Input: dimensioned drawing with shaded views. Units: mm. Origin: part minimum x, y, z. Give positions to 0.01 mm unless a question says otherwise; leave off trailing zeros. Order: outer loops, then holes, each group sorted by start corner. A loop starts at its lowest first (then second) coordinate and runs counter-clockwise, first axis right, second up. Notation, with made-up numbers: (70, -4.75) - (106, -4.75) arc R14 ccw to (106, 5.25) - close; hole circle Ø4 at (11.5, 39). An arc over 180 degrees is marked (long way). Use a Markdown table: item, result.
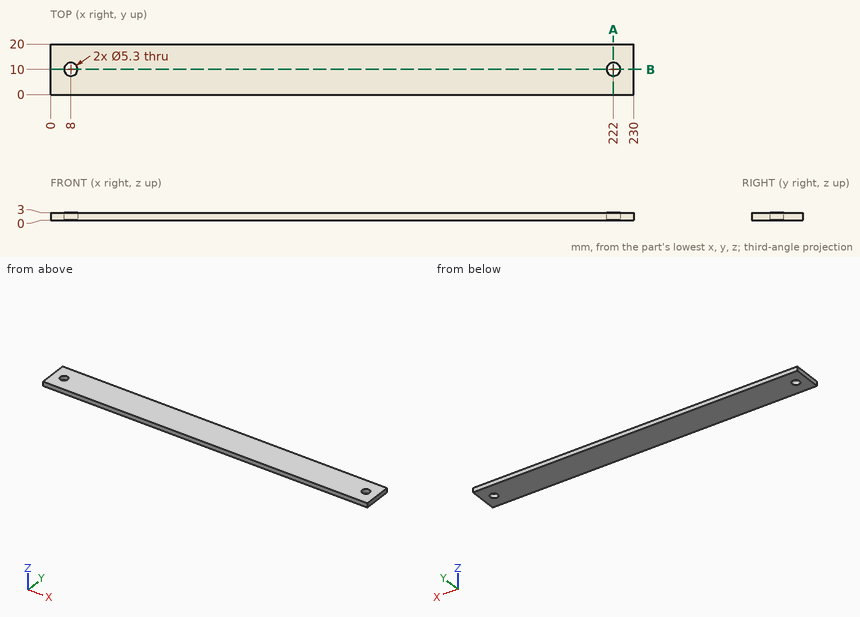
1. Section query B-B (y = 10). Return loops of the section in (x, z), then the cut area to 3 significant figures.
Response:
| item | result |
|---|---|
| outline | (0, 0) - (5.35, 0) - (5.35, 3) - (0, 3) - close; (10.65, 0) - (219.35, 0) - (219.35, 3) - (10.65, 3) - close; (224.65, 0) - (230, 0) - (230, 3) - (224.65, 3) - close |
| area | 658 mm^2 |
2. Section query A-A (x = 222). Return loops of the section in (y, z).
Response:
| item | result |
|---|---|
| outline | (0, 0) - (7.35, 0) - (7.35, 3) - (0, 3) - close; (12.65, 0) - (20, 0) - (20, 3) - (12.65, 3) - close |
3. Material intervals for line 1 along X through (y, z) = (10.25, 2.5); line 2 along Y through (x, z) = (222, 2.3); line 3 along X through (y, z) = (8.5, 1.4), sorted ascending.
Response:
| item | result |
|---|---|
| line 1 | x = 0 to 5.36, 10.64 to 219.36, 224.64 to 230 |
| line 2 | y = 0 to 7.35, 12.65 to 20 |
| line 3 | x = 0 to 5.82, 10.18 to 219.82, 224.18 to 230 |
4. Pin query (flat end, axial travel): pin 1 (2 mm diameter, centred on x = 204, y = 7.5, fed in from -Z); pin 2 (3 mm diameter, centred on x = 222, y = 10, fed in from +Z). Return the tip coordinate at first contact, or that it passes through.
Response:
| item | result |
|---|---|
| pin 1 | stops at z = 0 |
| pin 2 | passes through |
